```python
from build123d import *

# Parameters (mm, degrees)
F0_R     = 3.175
F1_DEPTH = 203.2
F2_R     = 12.7
F3_DEPTH = 6.35
F4_R     = 3.175
F5_DEPTH = 25.4


with BuildPart() as f1:
    # F0 (on Right) → F1 (new body, symmetric)
    with BuildSketch(Plane.YZ):
        Circle(F0_R)
    extrude(amount=F1_DEPTH, both=True)

    # F2 (on face) → F3 (join)
    with BuildSketch(Plane.YZ.offset(203.2)):
        Circle(F2_R)
    extrude(amount=F3_DEPTH)

    # F4 (on face) → F5 (join)
    with BuildSketch(Plane.YZ.offset(209.55)):
        with Locations((0, 7.846299)):
            Circle(F4_R)
    extrude(amount=F5_DEPTH)


solid = f1.part
```
Geometry check sheet. Reference: the model listing, model coordinates, mm. A direction names the side the tool comes from. Coordinates: 2 decimals unless noted, no trailing zeros. Order: outer loops, then holes, each group sorted by start corner. A loop starts at its lowest first (then second) coordinate and runs counter-clockwise, first axis right, second up. Notation, with made-up numbers: (87.25, 83.5) - (139.25, 83.5) arc R14 ccw to (139.25, 107.5) - close; hole circle Ø8 at (11.25, -15.75). An arc over 180 degrees is marked (long way). Answer as a JSON object with one key per item and string values. Group by question number.
Item 1: Depth check by flat-ended pin: pin 1 Ø4 at (x, z) = (-17, 2.5) entering from +Y; pin 2 Ø3 at (y, z) = (-10, -0.5) entering from +X; pin 3 Ø8 at (x, y) = (-43, -2) entering from -Z (3 decimals); pin 4 Ø6 at (x, z) = (-148.5, 6.5) entering from +Y. Enter the tip coordinate at first touch or a pass-through.
Item 2: Sectioned sample at A-A, the plane x = -66.5. Record the cut outline in (y, z) (3 decimals), and give its area (3 significant figures).
Item 3: Scan lines: probe 1 along X at (y, z) = (9.75, 2.5); probe 2 along Y at (x, z) = (160.5, -0.25); probe 3 along X at (y, z) = (-2.75, -0.25). Record each from-to range of solid material in increasing order.
Item 4: Tool access check on faces 1 (the face through (206.33, -2.75, -12.4)), 2 (the face through (203.2, 3, -3)). Record the directions out of +Z, -Z, +X, -X, +Y, -Y that give a thin tool (end or side, any length) a straight path to the whole face; none if there is none.
Resolved:
{
 "1": {"pin 1": "y = 3.14", "pin 2": "x = 209.55", "pin 3": "z = -3.175", "pin 4": "through"},
 "2": {"outline": "circle Ø6.35 at (0, 0)", "area": "31.7 mm^2"},
 "3": {"probe 1": "203.2 to 209.55", "probe 2": "-3.17 to 3.17", "probe 3": "-203.2 to 209.55"},
 "4": {"face 1": "+X, -X", "face 2": "-X"}
}
